Verification items for the finished model (mm, model axes). Coordinates: 2 decimals unless noted, no trailing zeros. Loops run counter-clockwise (first coordinate to the right, second up) from the corner with the lowest first, then second, coordinate; pieces in that order, holes last.
Q1. Material ranges on probe 1 along X at (y, z) = (-50, 1.2); probe 2 along Y at (x, z) = (-11, 0.5); probe 3 along Z at (x, y) = (12.5, -343), recorded low to high.
Q2. Sectioned sample at A-A (y = -228). Enter the section's corners in (x, z), then the cut area to 3 significant figures.
Q3. Go/stop test with flat-tipped pins: P1, Ø7, axis at x = 11, y = -450, coming from the +Z side; P2, Ø12, axis at x = 9, z = 5, coming from the +Y side; P3, Ø5, axis at x = -10, y = -127, coming from the +Z side; P4, Ø2, axis at y = -185.5, z = 14, coming from the -X side. Record where each tip stops, or that it passes through.
```python
from build123d import *

# Parameters (mm, degrees)
F1_W           = 9.8
F1_H           = 4
F1_W_2         = 12.4
F1_H_2         = 4.9
F3_DEPTH       = 500
F5_D           = 4.5
F5_CSINK_D     = 8
F5_CSINK_ANGLE = 90


with BuildPart() as f3:
    # F1 (on Front) → F3 (new body, through all)
    with BuildSketch(Plane.XZ):
        with Locations((11.1, 2)):
            Rectangle(F1_W, F1_H)
        Polygon((-6.2, 4), (-6.2, 0), (-4, 0), (-4, 3), (4, 3), (4, 0), (6.2, 0), (6.2, 4), align=None)
        with Locations((0, 6.45)):
            Rectangle(F1_W_2, F1_H_2)
        with BuildLine():
            ThreePointArc((5, 18), (-2.5739075352, 22.2866070499), (-2.35, 13.5866679255))
            ThreePointArc((-2.35, 13.5866679255), (0, 13), (2.35, 13.5866679255))
            ThreePointArc((2.35, 13.5866679255), (4.2866070499, 15.4260924648), (5, 18))
        make_face()
        with Locations((-11.1, 2)):
            Rectangle(F1_W, F1_H)
        with BuildLine():
            Line((-2.35, 13.5866679255), (-6.2, 8.9))
            Line((-6.2, 8.9), (6.2, 8.9))
            Line((6.2, 8.9), (2.35, 13.5866679255))
            ThreePointArc((2.35, 13.5866679255), (0, 13), (-2.35, 13.5866679255))
        make_face()
    extrude(amount=F3_DEPTH)

    # F5 (through all)
    with Locations(Plane.XY.offset(4)):
        with Locations((11, -50), (-11, -50), (-11, -150), (11, -150), (11, -250), (-11, -250), (11, -350), (-11, -350), (11, -450), (-11, -450)):
            CounterSinkHole(F5_D / 2, F5_CSINK_D / 2, counter_sink_angle=F5_CSINK_ANGLE)


with BuildPart() as f6_1:
    # F6: copy of F3
    add(f3.part)


solid = f3.part
```
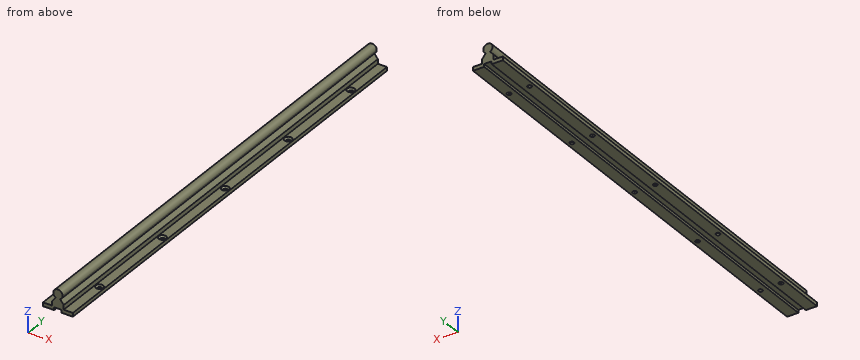
Geometry check:
1. probe 1: x = -16 to -13.25, -8.75 to -4, 4 to 8.75, 13.25 to 16
1. probe 2: y = -500 to -452.25, -447.75 to -352.25, -347.75 to -252.25, -247.75 to -152.25, -147.75 to -52.25, -47.75 to 0
1. probe 3: z = 0 to 4
2. outline: (-16, 0) - (-4, 0) - (-4, 3) - (4, 3) - (4, 0) - (16, 0) - (16, 4) - (6.2, 4) - (6.2, 8.9) - (2.35, 13.59) arc R5 ccw (long way) to (-2.35, 13.59) - (-6.2, 8.9) - (-6.2, 4) - (-16, 4) - close
2. area: 282 mm2
3. P1: stops at z = 3.5
3. P2: stops at y = 0
3. P3: stops at z = 4
3. P4: stops at x = -4
